```python
from build123d import *

# Parameters (mm, degrees)
F4_DEPTH = 9.907
F5_R     = 17.05
F5_R_2   = 15.9037
F5_R_3   = 13.9037
F5_R_4   = 12.9
F6_DEPTH = 1


with BuildPart() as f1:
    # F0 (on Front) → F1 (revolve)
    with BuildSketch(Plane.XZ):
        Polygon((0, 0), (0, 4.953), (-19.05, 4.953), (-19.05, 1.651), (-16.51, 1.651), (-16.51, 0), align=None)
        with BuildLine():
            Line((-16.51, 1.651), (-19.05, 1.651))
            add(Edge.make_bspline(
                [(-19.05, 1.651), (-17.78, 1.651), (-16.51, 0.8255), (-16.51, 0)],
                knots=[0, 0, 0, 0, 3.0294225522, 3.0294225522, 3.0294225522, 3.0294225522], degree=3))
            Line((-16.51, 0), (-16.51, 1.651))
        make_face()
    revolve(axis=Axis((0, 0, 11.7816049606), (0, 0, 1)))

    # F2: F1 across plane


with BuildPart() as f1_1:
    add(f1.part)
    add(f1.part.mirror(Plane.XY))

    # F3 (on face) → F4 (cut, through all)
    with BuildSketch(Plane.XY.offset(4.953)):
        with BuildLine():
            ThreePointArc((9.3683756747, -1.5759242424), (9.4670367304, -0.790705726), (9.5, 0))
            ThreePointArc((9.5, 0), (9.4670367304, 0.790705726), (9.3683756747, 1.5759242424))
            ThreePointArc((9.3683756747, 1.5759242424), (7.703557782, 2.5030376544), (8.5054801589, 4.2316435656))
            ThreePointArc((8.5054801589, 4.2316435656), (7.6856614466, 5.5839598968), (6.6528701021, 6.7815425534))
            ThreePointArc((6.6528701021, 6.7815425534), (4.7610605436, 6.5530376544), (4.3937803131, 8.4228673598))
            ThreePointArc((4.3937803131, 8.4228673598), (2.9356614466, 9.0350369048), (1.3961942733, 9.3968421053))
            ThreePointArc((1.3961942733, 9.3968421053), (0, 8.1), (-1.3961942733, 9.3968421053))
            ThreePointArc((-1.3961942733, 9.3968421053), (-2.9356614466, 9.0350369048), (-4.3937803131, 8.4228673598))
            ThreePointArc((-4.3937803131, 8.4228673598), (-4.2374363327, 8.068903265), (-4.1839598968, 7.6856614466))
            ThreePointArc((-4.1839598968, 7.6856614466), (-5.102542348, 6.371037111), (-6.6528701021, 6.7815425534))
            ThreePointArc((-6.6528701021, 6.7815425534), (-7.6856614466, 5.5839598968), (-8.5054801589, 4.2316435656))
            ThreePointArc((-8.5054801589, 4.2316435656), (-7.8728451297, 3.7162447399), (-7.6350369048, 2.9356614466))
            ThreePointArc((-7.6350369048, 2.9356614466), (-8.1709403471, 1.8341456097), (-9.3683756747, 1.5759242424))
            ThreePointArc((-9.3683756747, 1.5759242424), (-9.5, 0), (-9.3683756747, -1.5759242424))
            ThreePointArc((-9.3683756747, -1.5759242424), (-8.1709403471, -1.8341456097), (-7.6350369048, -2.9356614466))
            ThreePointArc((-7.6350369048, -2.9356614466), (-7.8728451297, -3.7162447399), (-8.5054801589, -4.2316435656))
            ThreePointArc((-8.5054801589, -4.2316435656), (-7.6856614466, -5.5839598968), (-6.6528701021, -6.7815425534))
            ThreePointArc((-6.6528701021, -6.7815425534), (-5.102542348, -6.371037111), (-4.1839598968, -7.6856614466))
            ThreePointArc((-4.1839598968, -7.6856614466), (-4.2374363327, -8.068903265), (-4.3937803131, -8.4228673598))
            ThreePointArc((-4.3937803131, -8.4228673598), (-2.9356614466, -9.0350369048), (-1.3961942733, -9.3968421053))
            ThreePointArc((-1.3961942733, -9.3968421053), (0, -8.1), (1.3961942733, -9.3968421053))
            ThreePointArc((1.3961942733, -9.3968421053), (2.9356614466, -9.0350369048), (4.3937803131, -8.4228673598))
            ThreePointArc((4.3937803131, -8.4228673598), (4.7610605436, -6.5530376544), (6.6528701021, -6.7815425534))
            ThreePointArc((6.6528701021, -6.7815425534), (7.6856614466, -5.5839598968), (8.5054801589, -4.2316435656))
            ThreePointArc((8.5054801589, -4.2316435656), (7.703557782, -2.5030376544), (9.3683756747, -1.5759242424))
        make_face()
        with BuildLine():
            ThreePointArc((8.5054801589, 4.2316435656), (7.703557782, 2.5030376544), (9.3683756747, 1.5759242424))
            ThreePointArc((9.3683756747, 1.5759242424), (9.0350369048, 2.9356614466), (8.5054801589, 4.2316435656))
        make_face()
        with BuildLine():
            ThreePointArc((8.5054801589, 4.2316435656), (9.0350369048, 2.9356614466), (9.3683756747, 1.5759242424))
            ThreePointArc((9.3683756747, 1.5759242424), (10.1365527417, 2.0715648888), (10.4350369048, 2.9356614466))
            ThreePointArc((10.4350369048, 2.9356614466), (9.8156201982, 4.0978532217), (8.5054801589, 4.2316435656))
        make_face()
        with BuildLine():
            ThreePointArc((10.4350369048, -2.9356614466), (10.1365527417, -2.0715648888), (9.3683756747, -1.5759242424))
            ThreePointArc((9.3683756747, -1.5759242424), (9.0350369048, -2.9356614466), (8.5054801589, -4.2316435656))
            ThreePointArc((8.5054801589, -4.2316435656), (9.8156201982, -4.0978532217), (10.4350369048, -2.9356614466))
        make_face()
        with BuildLine():
            ThreePointArc((8.5054801589, -4.2316435656), (9.0350369048, -2.9356614466), (9.3683756747, -1.5759242424))
            ThreePointArc((9.3683756747, -1.5759242424), (7.703557782, -2.5030376544), (8.5054801589, -4.2316435656))
        make_face()
        with BuildLine():
            ThreePointArc((4.3937803131, 8.4228673598), (4.7610605436, 6.5530376544), (6.6528701021, 6.7815425534))
            ThreePointArc((6.6528701021, 6.7815425534), (5.5839598968, 7.6856614466), (4.3937803131, 8.4228673598))
        make_face()
        with BuildLine():
            ThreePointArc((4.3937803131, 8.4228673598), (5.5839598968, 7.6856614466), (6.6528701021, 6.7815425534))
            ThreePointArc((6.6528701021, 6.7815425534), (6.8985842324, 7.2042438978), (6.9839598968, 7.6856614466))
            ThreePointArc((6.9839598968, 7.6856614466), (5.9672017152, 9.0321850106), (4.3937803131, 8.4228673598))
        make_face()
        with BuildLine():
            ThreePointArc((6.9839598968, -7.6856614466), (6.8985842324, -7.2042438978), (6.6528701021, -6.7815425534))
            ThreePointArc((6.6528701021, -6.7815425534), (5.5839598968, -7.6856614466), (4.3937803131, -8.4228673598))
            ThreePointArc((4.3937803131, -8.4228673598), (5.9672017152, -9.0321850106), (6.9839598968, -7.6856614466))
        make_face()
        with BuildLine():
            ThreePointArc((4.3937803131, -8.4228673598), (5.5839598968, -7.6856614466), (6.6528701021, -6.7815425534))
            ThreePointArc((6.6528701021, -6.7815425534), (4.7610605436, -6.5530376544), (4.3937803131, -8.4228673598))
        make_face()
        with BuildLine():
            ThreePointArc((-1.3961942733, 9.3968421053), (0, 8.1), (1.3961942733, 9.3968421053))
            ThreePointArc((1.3961942733, 9.3968421053), (0, 9.5), (-1.3961942733, 9.3968421053))
        make_face()
        with BuildLine():
            ThreePointArc((-1.3961942733, 9.3968421053), (0, 9.5), (1.3961942733, 9.3968421053))
            ThreePointArc((1.3961942733, 9.3968421053), (1.3990482448, 9.4483859641), (1.4, 9.5))
            ThreePointArc((1.4, 9.5), (-0.0516140359, 10.8990482448), (-1.3961942733, 9.3968421053))
        make_face()
        with BuildLine():
            ThreePointArc((1.4, -9.5), (1.3990482448, -9.4483859641), (1.3961942733, -9.3968421053))
            ThreePointArc((1.3961942733, -9.3968421053), (0, -9.5), (-1.3961942733, -9.3968421053))
            ThreePointArc((-1.3961942733, -9.3968421053), (-0.0516140359, -10.8990482448), (1.4, -9.5))
        make_face()
        with BuildLine():
            ThreePointArc((-1.3961942733, -9.3968421053), (0, -9.5), (1.3961942733, -9.3968421053))
            ThreePointArc((1.3961942733, -9.3968421053), (0, -8.1), (-1.3961942733, -9.3968421053))
        make_face()
        with BuildLine():
            ThreePointArc((-4.1839598968, 7.6856614466), (-4.2374363327, 8.068903265), (-4.3937803131, 8.4228673598))
            ThreePointArc((-4.3937803131, 8.4228673598), (-5.5839598968, 7.6856614466), (-6.6528701021, 6.7815425534))
            ThreePointArc((-6.6528701021, 6.7815425534), (-5.102542348, 6.371037111), (-4.1839598968, 7.6856614466))
        make_face()
        with BuildLine():
            ThreePointArc((-6.6528701021, 6.7815425534), (-5.5839598968, 7.6856614466), (-4.3937803131, 8.4228673598))
            ThreePointArc((-4.3937803131, 8.4228673598), (-6.40685925, 8.8182852387), (-6.6528701021, 6.7815425534))
        make_face()
        with BuildLine():
            ThreePointArc((-6.6528701021, -6.7815425534), (-6.40685925, -8.8182852387), (-4.3937803131, -8.4228673598))
            ThreePointArc((-4.3937803131, -8.4228673598), (-5.5839598968, -7.6856614466), (-6.6528701021, -6.7815425534))
        make_face()
        with BuildLine():
            ThreePointArc((-6.6528701021, -6.7815425534), (-5.5839598968, -7.6856614466), (-4.3937803131, -8.4228673598))
            ThreePointArc((-4.3937803131, -8.4228673598), (-4.2374363327, -8.068903265), (-4.1839598968, -7.6856614466))
            ThreePointArc((-4.1839598968, -7.6856614466), (-5.102542348, -6.371037111), (-6.6528701021, -6.7815425534))
        make_face()
        with BuildLine():
            ThreePointArc((-7.6350369048, 2.9356614466), (-7.8728451297, 3.7162447399), (-8.5054801589, 4.2316435656))
            ThreePointArc((-8.5054801589, 4.2316435656), (-9.0350369048, 2.9356614466), (-9.3683756747, 1.5759242424))
            ThreePointArc((-9.3683756747, 1.5759242424), (-8.1709403471, 1.8341456097), (-7.6350369048, 2.9356614466))
        make_face()
        with BuildLine():
            ThreePointArc((-9.3683756747, 1.5759242424), (-9.0350369048, 2.9356614466), (-8.5054801589, 4.2316435656))
            ThreePointArc((-8.5054801589, 4.2316435656), (-10.3665160276, 3.3682852387), (-9.3683756747, 1.5759242424))
        make_face()
        with BuildLine():
            ThreePointArc((-9.3683756747, -1.5759242424), (-10.3665160276, -3.3682852387), (-8.5054801589, -4.2316435656))
            ThreePointArc((-8.5054801589, -4.2316435656), (-9.0350369048, -2.9356614466), (-9.3683756747, -1.5759242424))
        make_face()
        with BuildLine():
            ThreePointArc((-9.3683756747, -1.5759242424), (-9.0350369048, -2.9356614466), (-8.5054801589, -4.2316435656))
            ThreePointArc((-8.5054801589, -4.2316435656), (-7.8728451297, -3.7162447399), (-7.6350369048, -2.9356614466))
            ThreePointArc((-7.6350369048, -2.9356614466), (-8.1709403471, -1.8341456097), (-9.3683756747, -1.5759242424))
        make_face()
    extrude(amount=-F4_DEPTH, mode=Mode.SUBTRACT)

    # F5 (on face) → F6 (cut)
    with BuildSketch(Plane(origin=(0, 0, -4.953), x_dir=(1, 0, 0), z_dir=(0, 0, -1))):
        Circle(F5_R)
        Circle(F5_R_2, mode=Mode.SUBTRACT)
        Circle(F5_R_3)
        Circle(F5_R_4, mode=Mode.SUBTRACT)
    extrude(amount=-F6_DEPTH, mode=Mode.SUBTRACT)


solid = f1_1.part
```
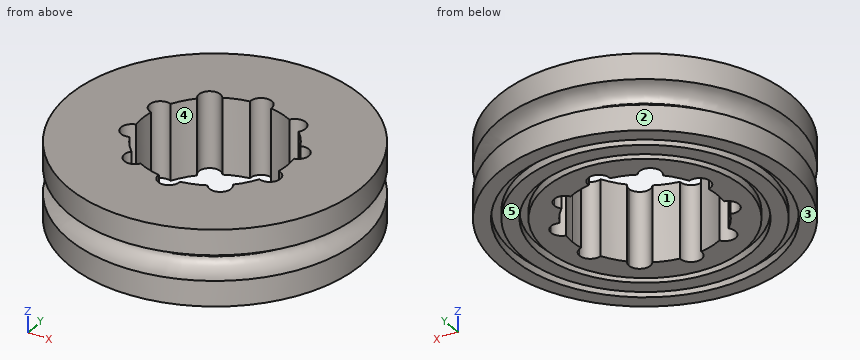
CAD build for the part. Positions are in the model's coordinates, mm. Face numbers are marked on the shaded views. A direction names the side the tool comes from. Coordinates: 2 decimals unless noted, no trailing zeros. Loops run counter-clockwise (first coordinate to the right, second up) from the corner with the lowest first, then second, coordinate; pieces in that order, holes last. Notation, with made-up numbers: (20, 50) - (58, 50) arc R31 cw to (58, 74) - close; hole circle Ø10 at (43, -7). An arc over 180 degrees is marked (long way). Use CSV: the item, a comma, the result in double quotes. Start each with the question number.
Q1. Probe probe 1 along Y at (x, z) = (0, -4.15); probe 2 along Z at (x, y) = (13, 3.5); probe 3 along X at (y, z) = (-1.5, -3). List the from-to ranges inside material, lowest first. Write a range as from..to.
Q2. 3-axis set-ups, long thin cutter, end or side, ignore diameter. For the marked faces 4 and 5: which of +Z, -Z, +X, -X, +Y, -Y reach the whole face in a straight line?
Q3. Cut at A-A, the plane z = 2.75. List the corners of the cut face in (x, y), then the cut area to 3 significant figures.
Q4. Drop flat-ended pins along their axis: P1, Ø1, axis at y = -4.5, z = 3.5, coming from the -X side; P2, Ø4, axis at x = 3, z = 2, coming from the +Y side; P3, Ø3, axis at x = -12.5, z = -2.5, coming from the -Y side. Give the stop position or say it passes through.
Q5. Two-plate mould, pull along X, no slides. Class the marked faces 1, 2 and 3: +X half, -X half, draft (parallel to the pull), parting line (faces both ways), or undercut.
Here are the results:
1,probe 1,"-19.05..-17.05, -15.9..-13.9, -12.9..-10.9, 10.9..12.9, 13.9..15.9, 17.05..19.05"
1,probe 2,"-3.95..4.95"
1,probe 3,"-18.99..-9.38, 9.38..18.99"
2,face 4,"+Z, -Z"
2,face 5,"-Z, +X, -X, +Y, -Y"
3,outline,"circle Ø38.1 at (0, 0); hole (-9.37, -1.58) arc R1.4 ccw (long way) to (-8.51, -4.23) arc R9.5 ccw to (-6.65, -6.78) arc R1.4 ccw (long way) to (-4.39, -8.42) arc R9.5 ccw to (-1.4, -9.4) arc R1.4 ccw (long way) to (1.4, -9.4) arc R9.5 ccw to (4.39, -8.42) arc R1.4 ccw (long way) to (6.65, -6.78) arc R9.5 ccw to (8.51, -4.23) arc R1.4 ccw (long way) to (9.37, -1.58) arc R9.5 ccw to (9.37, 1.58) arc R1.4 ccw (long way) to (8.51, 4.23) arc R9.5 ccw to (6.65, 6.78) arc R1.4 ccw (long way) to (4.39, 8.42) arc R9.5 ccw to (1.4, 9.4) arc R1.4 ccw (long way) to (-1.4, 9.4) arc R9.5 ccw to (-4.39, 8.42) arc R1.4 ccw (long way) to (-6.65, 6.78) arc R9.5 ccw to (-8.51, 4.23) arc R1.4 ccw (long way) to (-9.37, 1.58) arc R9.5 ccw to start"
3,area,"825 mm2"
4,P1,"x = -18.63"
4,P2,"y = 19.02"
4,P3,"y = -15.55"
5,face 1,"undercut"
5,face 2,"parting line"
5,face 3,"draft"
